Design review of the part built by this model. Coordinates are the model's own, in mm. Face numbers are marked on the shaded views. A direction names the side the tool comes from. Round coordinates to 2 decimals unless told otherwise and drop trailing zeros. Order: outer loops, then holes, each group sorted by start corner. A loop starts at its lowest first (then second) coordinate and runs counter-clockwise, first axis right, second up. Notation, with made-up numbers: (49.25, 23) - (69.25, 23) arc R3 cw to (69.25, 28) - close; hole circle Ø2 at (87.5, 61). An arc over 180 degrees is marked (long way). Answer as a JSON object with one key per item and string values. Group by question number.
from build123d import *

# Parameters (mm, degrees)
CROQUIS1_R              = 50
CROQUIS1_R_2            = 17.75
SALIENTE_EXTRUIR1_DEPTH = 70
CROQUIS2_R              = 40
CORTAR_EXTRUIR1_DEPTH   = 50
CROQUIS4_R              = 40
CROQUIS4_R_2            = 17.75
CORTAR_EXTRUIR3_DEPTH   = 10
CROQUIS5_R              = 2
CORTAR_EXTRUIR4_DEPTH   = 11
CROQUIS6_R              = 5
CORTAR_EXTRUIR5_DEPTH   = 5
REDONDEO2_R             = 1
CORTAR_EXTRUIR7_START   = -10
CROQUIS8_W              = 9
CROQUIS8_H              = 20
CORTAR_EXTRUIR7_DEPTH   = 4
CROQUIS9_R              = 52.339140615
CORTAR_EXTRUIR8_DEPTH   = 10
CROQUIS10_R             = 1.5
CORTAR_EXTRUIR9_DEPTH   = 30


with BuildPart() as part:
    # Croquis1 → Saliente-Extruir1 (new body)
    with BuildSketch(Plane.XY):
        Circle(CROQUIS1_R)
        Circle(CROQUIS1_R_2, mode=Mode.SUBTRACT)
    extrude(amount=SALIENTE_EXTRUIR1_DEPTH)

    # Croquis2 → Cortar-Extruir1 (cut)
    with BuildSketch(Plane.XY.offset(70)):
        Circle(CROQUIS2_R)
    extrude(amount=-CORTAR_EXTRUIR1_DEPTH, mode=Mode.SUBTRACT)

    # Croquis4 → Cortar-Extruir3 (cut)
    with BuildSketch(Plane.XY.offset(20)):
        Circle(CROQUIS4_R)
        with BuildLine():
            Line((-2.5, 27.386127875), (-2.5, 32.5))
            Line((-2.5, 32.5), (2.5, 32.5))
            Line((2.5, 32.5), (2.5, 27.386127875))
            ThreePointArc((2.5, 27.386127875), (19.445436483, 19.445436483), (27.386127875, 2.5))
            Line((27.386127875, 2.5), (32.5, 2.5))
            Line((32.5, 2.5), (32.5, -2.5))
            Line((32.5, -2.5), (27.386127875, -2.5))
            ThreePointArc((27.386127875, -2.5), (19.445436483, -19.445436483), (2.5, -27.386127875))
            Line((2.5, -27.386127875), (2.5, -32.5))
            Line((2.5, -32.5), (-2.5, -32.5))
            Line((-2.5, -32.5), (-2.5, -27.386127875))
            ThreePointArc((-2.5, -27.386127875), (-19.445436483, -19.445436483), (-27.386127875, -2.5))
            Line((-27.386127875, -2.5), (-32.5, -2.5))
            Line((-32.5, -2.5), (-32.5, 2.5))
            Line((-32.5, 2.5), (-27.386127875, 2.5))
            ThreePointArc((-27.386127875, 2.5), (-19.445436483, 19.445436483), (-2.5, 27.386127875))
        make_face(mode=Mode.SUBTRACT)
        with BuildLine():
            Line((-2.5, 22.5), (-2.5, 27.386127875))
            ThreePointArc((-2.5, 27.386127875), (-19.445436483, 19.445436483), (-27.386127875, 2.5))
            Line((-27.386127875, 2.5), (-22.5, 2.5))
            Line((-22.5, 2.5), (-22.5, -2.5))
            Line((-22.5, -2.5), (-27.386127875, -2.5))
            ThreePointArc((-27.386127875, -2.5), (-19.445436483, -19.445436483), (-2.5, -27.386127875))
            Line((-2.5, -27.386127875), (-2.5, -22.5))
            Line((-2.5, -22.5), (2.5, -22.5))
            Line((2.5, -22.5), (2.5, -27.386127875))
            ThreePointArc((2.5, -27.386127875), (19.445436483, -19.445436483), (27.386127875, -2.5))
            Line((27.386127875, -2.5), (22.5, -2.5))
            Line((22.5, -2.5), (22.5, 2.5))
            Line((22.5, 2.5), (27.386127875, 2.5))
            ThreePointArc((27.386127875, 2.5), (19.445436483, 19.445436483), (2.5, 27.386127875))
            Line((2.5, 27.386127875), (2.5, 22.5))
            Line((2.5, 22.5), (-2.5, 22.5))
        make_face()
        Circle(CROQUIS4_R_2, mode=Mode.SUBTRACT)
    extrude(amount=-CORTAR_EXTRUIR3_DEPTH, mode=Mode.SUBTRACT)

    # Croquis5 → Cortar-Extruir4 (cut, through all)
    with BuildSketch(Plane.XY.offset(10)):
        with Locations((21.213203436, 21.213203436)):
            Circle(CROQUIS5_R)
        with Locations((21.213203436, -21.213203436)):
            Circle(CROQUIS5_R)
        with Locations((-21.213203436, -21.213203436)):
            Circle(CROQUIS5_R)
        with Locations((-21.213203436, 21.213203436)):
            Circle(CROQUIS5_R)
    extrude(amount=-CORTAR_EXTRUIR4_DEPTH, mode=Mode.SUBTRACT)

    # Croquis6 → Cortar-Extruir5 (cut)
    with BuildSketch(Plane(origin=(0, 0, 0), x_dir=(-1, 0, 0), z_dir=(0, 0, -1))):
        with Locations((-21.213203436, 21.213203436)):
            Circle(CROQUIS6_R)
        with Locations((21.486974797, 21.486974797)):
            Circle(CROQUIS6_R)
        with Locations((21.760746158, -21.213203436)):
            Circle(CROQUIS6_R)
        with Locations((-20.939432074, -21.486974797)):
            Circle(CROQUIS6_R)
    extrude(amount=-CORTAR_EXTRUIR5_DEPTH, mode=Mode.SUBTRACT)

    # Redondeo2
    redondeo2_edges = [part.edges().sort_by_distance(p)[0] for p in [
        (-40, 0, 70),
        (-22.5, 0, 20),
        (2.5, -27.5, 20),
        (32.5, 0, 20),
        (27.5, 2.5, 20),
        (-2.5, 27.5, 20),
        (-27.5, -2.5, 20),
        (0, -22.5, 20),
        (0, 22.5, 20),
        (2.5, 27.5, 20),
        (0, 32.5, 20),
        (27.5, -2.5, 20),
        (22.5, 0, 20),
        (-2.5, -27.5, 20),
        (0, -32.5, 20),
        (-32.5, 0, 20),
        (-27.5, 2.5, 20),
        (-50, 0, 70),
    ]]
    fillet(redondeo2_edges, radius=REDONDEO2_R)

    # Croquis8 → Cortar-Extruir7 (cut)
    with BuildSketch(Plane.XY.offset(70).offset(CORTAR_EXTRUIR7_START)):
        with Locations((0, 45)):
            Rectangle(CROQUIS8_W, CROQUIS8_H)
    extrude(amount=-CORTAR_EXTRUIR7_DEPTH, mode=Mode.SUBTRACT)

    # Croquis9 → Cortar-Extruir8 (cut)
    with BuildSketch(Plane.XY.offset(70)):
        Circle(CROQUIS9_R)
    extrude(amount=-CORTAR_EXTRUIR8_DEPTH, mode=Mode.SUBTRACT)

    # Croquis10 → Cortar-Extruir9 (cut)
    with BuildSketch(Plane.XY.offset(60)):
        with Locations((31.819805153, 31.819805153)):
            Circle(CROQUIS10_R)
        with Locations((31.819805153, -31.819805153)):
            Circle(CROQUIS10_R)
        with Locations((-31.819805153, -31.819805153)):
            Circle(CROQUIS10_R)
        with Locations((-31.819805153, 31.819805153)):
            Circle(CROQUIS10_R)
    extrude(amount=-CORTAR_EXTRUIR9_DEPTH, mode=Mode.SUBTRACT)


solid = part.part
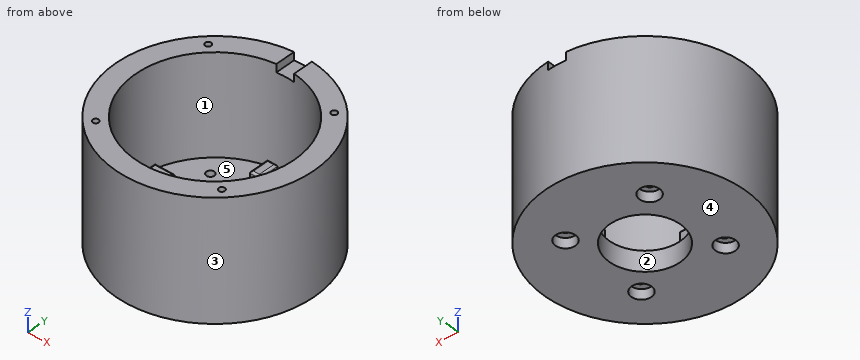
1. Mouldability with a two-part tool opening along X and no side actions: class the marked faces 3, 4 and 5 as pulls with the +X half, pulls with the -X half, needs draft (parallel to the pull), parting line crosses it, or undercut.
2. To check wall thickness, follow line 1 (Z direction, x = 24, y = -15); line 2 (Z direction, x = 0, y = 43.5); line 3 (Y direction, x = 6.5, z = 39). State the ranges of each line that lie inside material, in increasing order. Write a range as from..to.
3. Take a section at A-A, the plane z = 12.5. Give the boundary of the cut face in (x, y), then the cut area to 3 significant figures.
4. Clearance check with flat-ended pins moving along their axes: P1, Ø5.5, axis at y = -1, z = 13, coming from the -X side; P2, Ø10, axis at x = -14.5, z = 47.5, coming from the -Y side; P3, Ø1.5, axis at x = 0, z = 15.5, coming from the -Y side; P4, Ø8, axis at x = -27.5, z = 32, coming from the -Y side. State where each tip first meets the part, or that it passes through.
5. Take a section at C-C, the plane y = 0. Give the boundary of the cut face in (x, z), then the cut area to 3 significant figures.
6. Tool access review of the marked faces 1 and 2: name each direction out of +Z, -Z, +X, -X, +Y, -Y from which nothing blocks a thin tool from reaching the whole face with its end or side.
7. Take a section at D-D, the plane x = -20.5. Give the boundary of the cut face in (y, z).
8. Take a section at B-B, the plane x = 0. Give the boundary of the cut face in (y, z).
Response values:
{
 "1": {"face 3": "parting line crosses it", "face 4": "needs draft", "face 5": "undercut"},
 "2": {"line 1": "0..10", "line 2": "0..56", "line 3": "-49.58..-39.47, 39.47..49.58"},
 "3": {"outline": "circle Ø100 at (0, 0); (-32.5, -2.5) - (-22.5, -2.5) - (-22.5, 2.5) - (-32.5, 2.5) - close; (-2.5, -32.5) - (2.5, -32.5) - (2.5, -22.5) - (-2.5, -22.5) - close; (-2.5, 22.5) - (2.5, 22.5) - (2.5, 32.5) - (-2.5, 32.5) - close; (22.5, -2.5) - (32.5, -2.5) - (32.5, 2.5) - (22.5, 2.5) - close; hole circle Ø80 at (0, 0)", "area": "3,030 mm2"},
 "4": {"P1": "x = -50", "P2": "y = -49.09", "P3": "y = -50", "P4": "y = -44.13"},
 "5": {"outline": "(-50, 0) - (-17.75, 0) - (-17.75, 10) - (-22.5, 10) - (-22.5, 19) arc R1 ccw to (-23.5, 20) - (-31.5, 20) arc R1 ccw to (-32.5, 19) - (-32.5, 10) - (-40, 10) - (-40, 60) - (-50, 60) - close; (17.75, 0) - (50, 0) - (50, 60) - (40, 60) - (40, 10) - (32.5, 10) - (32.5, 19) arc R1 ccw to (31.5, 20) - (23.5, 20) arc R1 ccw to (22.5, 19) - (22.5, 10) - (17.75, 10) - close", "area": "1,840 mm2"},
 "6": {"face 1": "+Z", "face 2": "+Z, -Z"},
 "7": {"outline": "(-45.6, 0) - (-26.05, 0) - (-26.05, 5) - (-23.08, 5) - (-23.08, 10) - (-34.35, 10) - (-34.35, 60) - (-45.6, 60) - close; (-19.34, 5) - (-16.37, 5) - (-16.37, 0) - (16.59, 0) - (16.59, 5) - (19.34, 5) - (19.34, 10) - (-19.34, 10) - close; (23.08, 5) - (26.39, 5) - (26.39, 0) - (45.6, 0) - (45.6, 60) - (34.35, 60) - (34.35, 10) - (23.08, 10) - close"},
 "8": {"outline": "(-50, 0) - (-17.75, 0) - (-17.75, 10) - (-22.5, 10) - (-22.5, 19) arc R1 ccw to (-23.5, 20) - (-31.5, 20) arc R1 ccw to (-32.5, 19) - (-32.5, 10) - (-40, 10) - (-40, 60) - (-50, 60) - close; (17.75, 0) - (50, 0) - (50, 56) - (40, 56) - (40, 10) - (32.5, 10) - (32.5, 19) arc R1 ccw to (31.5, 20) - (23.5, 20) arc R1 ccw to (22.5, 19) - (22.5, 10) - (17.75, 10) - close"}
}
